Source: CAD feature listing. Evaluate the final solid. Frame: model axes, mm. Face numbers are marked on the shaded views. A direction names the side the tool comes from. Round coordinates to 2 decimals unless told otherwise and drop trailing zeros. Write each loop counter-clockwise with the first axis right and the second up, starting at its lowest first coordinate (ties: lowest second). Pieces come first, ordered by that corner, then holes. Notation, with made-up numbers: M 9.25,45.25 L 28.25,45.25 A8 ccw 28.25,60.25 Z; hole C 70.25,16.25 d11. An arc over 180 degrees is marked long. Put each result on its own line as item: value. Start each with the question number.
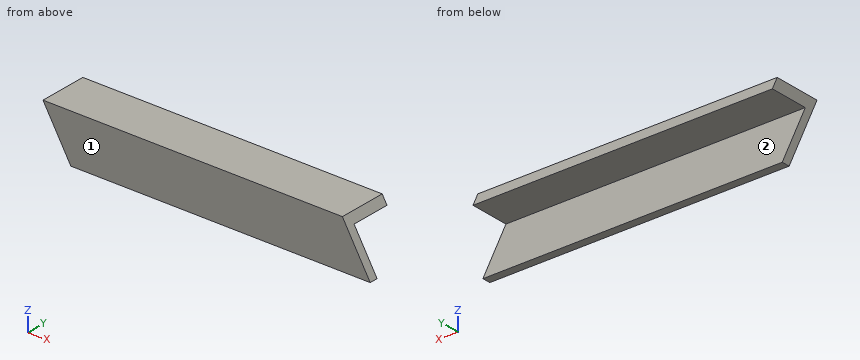
```python
from build123d import *

# Parameters (mm, degrees)
BOSS_EXTRUDE1_DEPTH = 240
CUT_EXTRUDE1_DEPTH  = 242.660919472


with BuildPart() as part:
    # Sketch1 → Boss-Extrude1 (new body)
    with BuildSketch(Plane(origin=(0, 0, 0), x_dir=(0, 0, -1), z_dir=(1, 0, 0))):
        Polygon((0, 0), (20, 0), (20, 3.461178467), (3.461178467, 3.461178467), (3.461178467, 20), (0, 20), align=None)
    extrude(amount=BOSS_EXTRUDE1_DEPTH)

    # Sketch2 → Cut-Extrude1 (cut, through all)
    with BuildSketch(Plane.XZ):
        Polygon((0, 0), (11.547005384, -20), (0, -20), align=None)
        Polygon((240, 0), (240, -20), (135.67731326, -20), (124.130307876, 0), align=None)
    extrude(amount=-CUT_EXTRUDE1_DEPTH, mode=Mode.SUBTRACT)


solid = part.part
```
(1) Section query C-C (z = -6.5). Return loops of the section in (x, y), and give its area (3 significant figures).
(2) Section query B-B (y = 18.75). Return loops of the section in (x, z).
(3) Contact query for flat-ended pins moving along their axis: P1, Ø8, axis at x = 28, z = -5.5, coming from the +Y side; P2, Ø1.5, axis at x = 73, y = 9.5, coming from the -Z side; P3, Ø5, axis at x = 35.5, z = -14.5, coming from the +Y side. Output: stop coordinate, or through.
(4) Section query A-A (x = 43). Return loops of the section in (y, z).
(5) Ray query, line 1 along Z through (x, y) = (45.5, 6); line 2 along Y through (x, z) = (110.5, -6.5). Return the intervals inside material, ascending.
(6) Access query for the marked faces 1 and 2. Directions: +Z, -Z, +X, -X, +Y, -Y. A direction counts if a zero-diameter tool reaches every point of the face in a straight line with its end or side. Return the directions, or none.
Entries:
1. outline: M 3.75,0 L 127.88,0 L 127.88,3.46 L 3.75,3.46 Z
1. area: 430 mm2
2. outline: M 0,0 L 2,-3.46 L 126.13,-3.46 L 124.13,0 Z
3. P1: y = 20
3. P2: z = -3.46
3. P3: y = 3.46
4. outline: M 0,-20 L 3.46,-20 L 3.46,-3.46 L 20,-3.46 L 20,0 L 0,0 Z
5. line 1: -3.46 to 0
5. line 2: 0 to 3.46
6. face 1: +Z, -Z, +X, -X, -Y
6. face 2: -Z, +X, -X, +Y
